```python
from build123d import *

# Parameters (mm, degrees)
SKETCH1_R            = 39
EXTRUDE1_DEPTH       = 2
SKETCH2_R            = 26
EXTRUDE3_DEPTH       = 15
FILLET1_R            = 1
SHELL1_OUTLINE_R     = 24
SHELL1_DEPTH         = 15
FILLET3_R            = 0.2
FILLET4_R            = 0.5
FILLET5_R            = 1
M5_CLEARANCE_HOLE2_D = 5.3
CIRPATTERN2_COUNT    = 4
EXTRUDE4_DEPTH       = 0.5


# Read off the part's stored shape, not the designer's step: Shell1
with BuildPart() as part:
    # Sketch1 → Extrude1 (new body)
    with BuildSketch(Plane.XY):
        Circle(SKETCH1_R)
    extrude(amount=EXTRUDE1_DEPTH)

    # Sketch2 → Extrude3 (add)
    with BuildSketch(Plane.XY.offset(2)):
        Circle(SKETCH2_R)
    extrude(amount=EXTRUDE3_DEPTH)

    # Fillet1
    fillet1_edges = [part.edges().sort_by_distance(p)[0] for p in [
        (-26, 0, 17),
    ]]
    fillet(fillet1_edges, radius=FILLET1_R)

    # Shell1 outline → Shell1 (cut)
    with BuildSketch(Plane.XY):
        Circle(SHELL1_OUTLINE_R)
    extrude(amount=SHELL1_DEPTH, mode=Mode.SUBTRACT)

    # Fillet3
    fillet3_edges = [part.edges().sort_by_distance(p)[0] for p in [
        (-26, 0, 2),
    ]]
    fillet(fillet3_edges, radius=FILLET3_R)

    # Fillet4
    fillet4_edges = [part.edges().sort_by_distance(p)[0] for p in [
        (-24, 0, 0),
    ]]
    fillet(fillet4_edges, radius=FILLET4_R)

    # Fillet5
    fillet5_edges = [part.edges().sort_by_distance(p)[0] for p in [
        (-24, 0, 15),
    ]]
    fillet(fillet5_edges, radius=FILLET5_R)

    # M5 Clearance Hole2 (through all)
    with Locations(Plane.XY.offset(2)):
        with Locations((0, 32.5)):
            m5_clearance_hole2 = Hole(M5_CLEARANCE_HOLE2_D / 2)

    # CirPattern2: M5 Clearance Hole2 ×4 about axis
    cirpattern2_axis = Axis((0, 0, 0), (0, 0, 1))
    for i in range(1, CIRPATTERN2_COUNT):
        add(m5_clearance_hole2.rotate(cirpattern2_axis, i * 360 / CIRPATTERN2_COUNT), mode=Mode.SUBTRACT)

    # Sketch7 → Extrude4 (add)
    # profile 1 of 5: a face of its own
    with BuildSketch(Plane.XY.offset(17)):
        with BuildLine():
            Line((19.676957621, 5.895197773), (19.909210058, 4.601855926))
            add(Edge.make_bspline(
                [(19.909210058, 4.601855926), (19.926651632, 4.500756414), (19.960375824, 4.305275227), (20.003127109, 4.021131614), (20.035136253, 3.755856277), (20.057801947, 3.50941192), (20.070613778, 3.281967505), (20.074435398, 3.073479481), (20.066961458, 2.884011603), (20.051245996, 2.710939809), (20.024412986, 2.550248712), (19.989932757, 2.397223976), (19.945515818, 2.249766305), (19.894274619, 2.106997056), (19.832166687, 1.970108117), (19.761460303, 1.838667258), (19.682767862, 1.711818388), (19.595037947, 1.5917147), (19.499748057, 1.479638905), (19.396983344, 1.377993746), (19.28704005, 1.288275306), (19.170652181, 1.209353696), (19.046580749, 1.143616013), (18.91635037, 1.087389919), (18.77889519, 1.043285188), (18.68385402, 1.023944482), (18.635902767, 1.014186489)],
                knots=[0, 0, 0, 0, 1.730076892, 3.345194012, 4.845031028, 6.235470528, 7.517952796, 8.685973408, 9.750415481, 10.714141801, 11.614495518, 12.495817449, 13.357576408, 14.209987726, 15.051935834, 15.889834422, 16.725466702, 17.567259816, 18.395636046, 19.203792226, 20.001166367, 20.785517328, 21.571153748, 22.36530307, 23.175244092, 24, 24, 24, 24], degree=3))
            add(Edge.make_bspline(
                [(18.635902767, 1.014186489), (18.601332211, 1.008792177), (18.532676771, 0.998079338), (18.429279177, 0.989999215), (18.326869474, 0.989175032), (18.22517881, 0.995885426), (18.124571089, 1.010143405), (18.024571455, 1.030831771), (17.925656818, 1.059215457), (17.827998765, 1.094745096), (17.732265048, 1.137285173), (17.638741204, 1.185398285), (17.548021241, 1.239670585), (17.460576449, 1.300003798), (17.375273895, 1.365504104), (17.293439096, 1.437570028), (17.213363047, 1.514802593), (17.112225961, 1.626941287), (16.993341681, 1.77534263), (16.86772283, 1.966533878), (16.757516889, 2.168158053), (16.678159583, 2.347681675), (16.62103193, 2.506628847), (16.578084306, 2.647799896), (16.532403009, 2.80962355), (16.487908625, 2.993283627), (16.441312375, 3.197882505), (16.392833179, 3.423332012), (16.345041361, 3.670140713), (16.313480153, 3.841752829), (16.297053942, 3.931069335)],
                knots=[0, 0, 0, 0, 0.700069007, 1.390302967, 2.07345339, 2.748157948, 3.427928198, 4.105586319, 4.790313218, 5.485605459, 6.183746622, 6.885581077, 7.589368078, 8.297874576, 9.010777227, 9.740496332, 10.479143782, 11.236028141, 12.761351436, 14.279847751, 15.808380735, 17.355454046, 18.202580936, 19.187428998, 20.308031537, 21.567474943, 22.968881258, 24.507767656, 26.182447736, 28, 28, 28, 28], degree=3))
            Line((16.297053942, 3.931069335), (16.061091402, 5.244445737))
            Line((16.061091402, 5.244445737), (19.676957621, 5.895197773))
        make_face()
        with BuildLine():
            Line((19.208000623, 4.688672333), (16.929997485, 4.27833496))
            Line((16.929997485, 4.27833496), (17.021266015, 3.771534913))
            add(Edge.make_bspline(
                [(17.021266015, 3.771534913), (17.032345987, 3.711373225), (17.053733, 3.595246685), (17.089409635, 3.428546915), (17.125904798, 3.275194319), (17.162274443, 3.135102557), (17.201293405, 3.00858141), (17.239805196, 2.895047806), (17.280674034, 2.795284581), (17.322803022, 2.707562492), (17.367167925, 2.628795417), (17.415768928, 2.556722787), (17.467747655, 2.489006687), (17.5235422, 2.425554712), (17.583554861, 2.366990452), (17.647740166, 2.313415224), (17.715443468, 2.264358919), (17.78654117, 2.219690581), (17.86093744, 2.180915018), (17.938988478, 2.150582726), (18.019080747, 2.126625083), (18.101820962, 2.110326722), (18.187002339, 2.10138524), (18.27462071, 2.100115904), (18.364754991, 2.105817523), (18.424984256, 2.11557869), (18.455591769, 2.120539153)],
                knots=[0, 0, 0, 0, 1.775092123, 3.426355128, 4.946159467, 6.349362224, 7.625332135, 8.787500866, 9.827139712, 10.751664961, 11.609871591, 12.447943051, 13.271974121, 14.085592912, 14.897690682, 15.702716349, 16.509563741, 17.322105437, 18.137463576, 18.939829159, 19.748303036, 20.560495954, 21.383244435, 22.230303678, 23.100669685, 24, 24, 24, 24], degree=3))
            add(Edge.make_bspline(
                [(18.455591769, 2.120539153), (18.501912095, 2.1305263), (18.592653852, 2.150091173), (18.721035792, 2.198320249), (18.838930231, 2.260006867), (18.945420071, 2.337235377), (19.040204715, 2.429694213), (19.124665474, 2.535983583), (19.198010124, 2.656956303), (19.236010853, 2.745299303), (19.255489939, 2.790583724)],
                knots=[0, 0, 0, 0, 1.038177342, 2.033794765, 2.997232208, 3.948913134, 4.908064258, 5.892578705, 6.919740629, 8, 8, 8, 8], degree=3))
            add(Edge.make_bspline(
                [(19.255489939, 2.790583724), (19.271340372, 2.835554425), (19.304366828, 2.929256779), (19.335515387, 3.082108884), (19.356237644, 3.249799018), (19.363578257, 3.433371754), (19.359499759, 3.632545511), (19.343394445, 3.847458387), (19.316080336, 4.078281915), (19.288886141, 4.236399757), (19.274782474, 4.31840407)],
                knots=[0, 0, 0, 0, 0.739780208, 1.541429103, 2.416204183, 3.362112403, 4.391764505, 5.508663336, 6.707923483, 8, 8, 8, 8], degree=3))
            Line((19.274782474, 4.31840407), (19.208000623, 4.688672333))
        make_face(mode=Mode.SUBTRACT)
    # profile 2 of 5: a face of its own
    with BuildSketch(Plane.XY.offset(17)):
        Polygon((17.581435301, 10.747395777), (19.049151981, 7.917329337), (18.439211075, 7.601228576), (17.479778483, 9.451827868), (16.887646071, 9.144631354), (17.847078663, 7.294032062), (17.248268066, 6.983867465), (16.288835474, 8.834466757), (15.427349597, 8.388512397), (16.386782189, 6.537913105), (15.774615222, 6.220328302), (14.306898542, 9.050394742), align=None)
    # profile 3 of 5: a face of its own
    with BuildSketch(Plane.XY.offset(17)):
        Polygon((12.123844788, 16.457580555), (12.917806794, 15.714817969), (12.143879344, 12.912948311), (14.90345383, 13.856798471), (15.686285527, 13.124424172), (13.88243353, 9.757134842), (13.100343854, 10.488767121), (14.234893299, 12.619108166), (11.735026012, 11.766526536), (11.018976165, 12.436571107), (11.715733477, 14.975765485), (9.656626406, 13.71136244), (8.865632482, 14.451156944), align=None)
    # profile 4 of 5: a face of its own
    with BuildSketch(Plane.XY.offset(17)):
        with BuildLine():
            Line((5.883258698, 19.717752428), (6.913183244, 19.299994849))
            Line((6.913183244, 19.299994849), (6.01756442, 17.092483664))
            add(Edge.make_bspline(
                [(6.01756442, 17.092483664), (6.008486233, 17.069548786), (5.990944466, 17.025231756), (5.968459411, 16.960233961), (5.951756013, 16.899082481), (5.937700658, 16.842866609), (5.929563581, 16.790459558), (5.925628424, 16.742326117), (5.926160317, 16.698062126), (5.932981546, 16.644156349), (5.953878485, 16.579582514), (5.992366342, 16.504378403), (6.046995799, 16.430571608), (6.116233762, 16.35835831), (6.199026795, 16.288695912), (6.296204469, 16.225423966), (6.404381617, 16.164332538), (6.483415994, 16.131018738), (6.524364467, 16.113758537)],
                knots=[0, 0, 0, 0, 0.923038225, 1.783585378, 2.571857434, 3.294764068, 3.950625969, 4.554034933, 5.100209756, 5.604208717, 6.582094882, 7.621105052, 8.754146159, 10.004648243, 11.358032571, 12.793050822, 14.338448695, 16, 16, 16, 16], degree=3))
            add(Edge.make_bspline(
                [(6.524364467, 16.113758537), (6.568381949, 16.096937583), (6.653613085, 16.064367136), (6.781720621, 16.029178008), (6.904523521, 16.008154167), (7.020730873, 16.000176227), (7.127582444, 16.005957413), (7.223056232, 16.022459059), (7.306086108, 16.050112017), (7.366327548, 16.0847227), (7.408808112, 16.121187462), (7.440283212, 16.156538569), (7.473227208, 16.198887508), (7.50531201, 16.249796421), (7.539045, 16.307675031), (7.572073799, 16.374126456), (7.606128878, 16.448155364), (7.628152069, 16.500530119), (7.639621378, 16.527806013)],
                knots=[0, 0, 0, 0, 1.618793555, 3.134473113, 4.557098125, 5.894372325, 7.128811318, 8.225928628, 9.215199246, 10.122001872, 10.59222323, 11.133722231, 11.745813266, 12.4342968, 13.199761712, 14.047507939, 14.983174849, 16, 16, 16, 16], degree=3))
            Line((7.639621378, 16.527806013), (8.502591297, 18.654436956))
            Line((8.502591297, 18.654436956), (9.532515842, 18.235937357))
            Line((9.532515842, 18.235937357), (8.707388973, 16.202058985))
            add(Edge.make_bspline(
                [(8.707388973, 16.202058985), (8.690264857, 16.160919945), (8.657399682, 16.081964525), (8.607108499, 15.969669644), (8.55744861, 15.868768385), (8.509112965, 15.77872354), (8.462814268, 15.699035754), (8.416936123, 15.630448533), (8.37187755, 15.573021449), (8.326805301, 15.525418292), (8.279703663, 15.484600977), (8.228647973, 15.447875675), (8.172850214, 15.413626493), (8.111856943, 15.382432709), (8.046190439, 15.352664304), (7.974955261, 15.326194129), (7.898819327, 15.302555845), (7.790866987, 15.273622216), (7.649377033, 15.247349008), (7.474537056, 15.230788837), (7.294493017, 15.231346738), (7.108853114, 15.247073838), (6.916109728, 15.279574202), (6.715415009, 15.329190125), (6.505627921, 15.395521078), (6.364781141, 15.450317186), (6.29211203, 15.478588933)],
                knots=[0, 0, 0, 0, 1.100735908, 2.112569176, 3.038882457, 3.878101929, 4.636766245, 5.314609658, 5.914814222, 6.437739277, 6.931472359, 7.452107952, 7.989676895, 8.547154927, 9.143334263, 9.769772578, 10.422934341, 11.112083662, 12.529703976, 13.971813743, 15.444304845, 16.971076327, 18.569180017, 20.267430496, 22.074201565, 24, 24, 24, 24], degree=3))
            add(Edge.make_bspline(
                [(6.29211203, 15.478588933), (6.244182676, 15.498433981), (6.149939842, 15.53745503), (6.013814463, 15.602683122), (5.88435309, 15.670306438), (5.761925489, 15.742097212), (5.646414389, 15.816675017), (5.537586093, 15.894793889), (5.435720867, 15.976466149), (5.341250196, 16.061358864), (5.25487038, 16.147851514), (5.176741706, 16.233925948), (5.107139964, 16.319311849), (5.047198038, 16.404936156), (4.994627838, 16.489150823), (4.952167889, 16.573792183), (4.917824859, 16.65753338), (4.891447957, 16.742475337), (4.875614972, 16.831896812), (4.870930006, 16.928509796), (4.876515247, 17.033590153), (4.892769381, 17.147072804), (4.917918785, 17.269428531), (4.955303193, 17.399827213), (5.000827179, 17.539834697), (5.038531814, 17.63460801), (5.058131828, 17.683874055)],
                knots=[0, 0, 0, 0, 1.280434306, 2.517700506, 3.724934716, 4.885287436, 6.020054073, 7.118151758, 8.190968479, 9.241662168, 10.251996506, 11.207382413, 12.110466848, 12.96936814, 13.786218001, 14.559020287, 15.303990097, 16.01869134, 16.7505329, 17.539379253, 18.401400366, 19.344393315, 20.3670884, 21.482635478, 22.691397491, 24, 24, 24, 24], degree=3))
            Line((5.058131828, 17.683874055), (5.883258698, 19.717752428))
        make_face()
    # profile 5 of 5: a face of its own
    with BuildSketch(Plane.XY.offset(17)):
        Polygon((1.522878641, 20.560870651), (2.626263223, 20.419144723), (2.243380611, 17.431769924), (3.852081199, 17.225488206), (3.767490854, 16.56286384), (1.055405684, 16.910871486), align=None)
    extrude(amount=EXTRUDE4_DEPTH)


solid = part.part
```
Source: CAD feature listing. Evaluate the final solid. Frame: model axes, mm. A direction names the side the tool comes from. Round coordinates to 2 decimals unless told otherwise and drop trailing zeros. Write each loop counter-clockwise with the first axis right and the second up, starting at its lowest first coordinate (ties: lowest second). Pieces come first, ordered by that corner, then holes. Notation, with made-up numbers: M 5,84.25 L 58,84.25 A22 ccw 58,92.25 Z; hole C -18.5,2.25 d7. An arc over 180 degrees is marked long. Answer as a JSON object with one key per item and string values. Group by question number.
(1) Mould query, pull axis X, two halves, no side actions, for faces 3 (the flat face through (-1, 27, 2)), 4 (the cylindrical face through (-23.977, 1.055, 7.156)), 5 (the cylindrical face through (-5.077, 38.668, 0.986)). Classes: +X half, -X half, draft (parallel to the pull), parting line (faces both ways), or undercut.
(2) First-contact query: pin 1 (1 mm diameter, centred on x = -9, z = 7, fed in from -Y); pin 2 (0.7 mm diameter, centred on x = 18.5, y = 3, fed in from +Z); pin 3 (10 mm diameter, centred on x = -5.5, z = 3.5, fed in from -Y); pin 4 (4 mm diameter, centred on x = 32.5, y = 0, fed in from -Z). Flat tips, straight axial feed; report the tip coordinate or a pass-through.
(3) Ray query, line 1 (Y direction, x = 0, z = 0.7); line 2 (Z direction, x = -28, y = -6.5); line 3 (Z direction, x = -3.5, y = 4). Return the intervals inside material, ascending. Write a range as [from, to].
(4) Section query C-C on z = 10.75. Output: boundary loops of the cut face in (x, y).
(5) Reachability of faces 1 (the flat face through (13, 13, 17.5)), 2 (the flat face through (14.797, 11.464, 17.246)) from +Z, -Z, +X, -X, +Y, -Y: full face, straight path, thin tool, end or side. Return the list, or none.
(6) Section query D-D on x = 32.5. Output: boundary loops of the cut face in (y, z).
(7) Section query A-A on x = 0. Output: boundary loops of the cut face in (y, z), then the cut area to 3 significant figures.
Computed values:
{
 "1": {"face 3": "draft", "face 4": "undercut", "face 5": "parting line"},
 "2": {"pin 1": "y = -24.57", "pin 2": "z = 17", "pin 3": "y = -38.99", "pin 4": "through"},
 "3": {"line 1": "[-39, -35.15], [-29.85, -24], [24, 29.85], [35.15, 39]", "line 2": "[0, 2]", "line 3": "[15, 17]"},
 "4": {"outline": "C 0,0 d52; hole C 0,0 d48"},
 "5": {"face 1": "+Z, +X, -X, +Y, -Y", "face 2": "+Z"},
 "6": {"outline": "M -21.56,0 L -2.65,0 L -2.65,2 L -21.56,2 Z; M 2.65,0 L 21.56,0 L 21.56,2 L 2.65,2 Z"},
 "7": {"outline": "M -39,0 L -35.15,0 L -35.15,2 L -39,2 Z; M -29.85,0 L -24.5,0 A0.5 ccw -24,0.5 L -24,14 A1 cw -23,15 L 23,15 A1 cw 24,14 L 24,0.5 A0.5 ccw 24.5,0 L 29.85,0 L 29.85,2 L 26.2,2 A0.2 cw 26,2.2 L 26,16 A1 ccw 25,17 L -25,17 A1 ccw -26,16 L -26,2.2 A0.2 cw -26.2,2 L -29.85,2 Z; M 35.15,0 L 39,0 L 39,2 L 35.15,2 Z", "area": "195 mm^2"}
}
